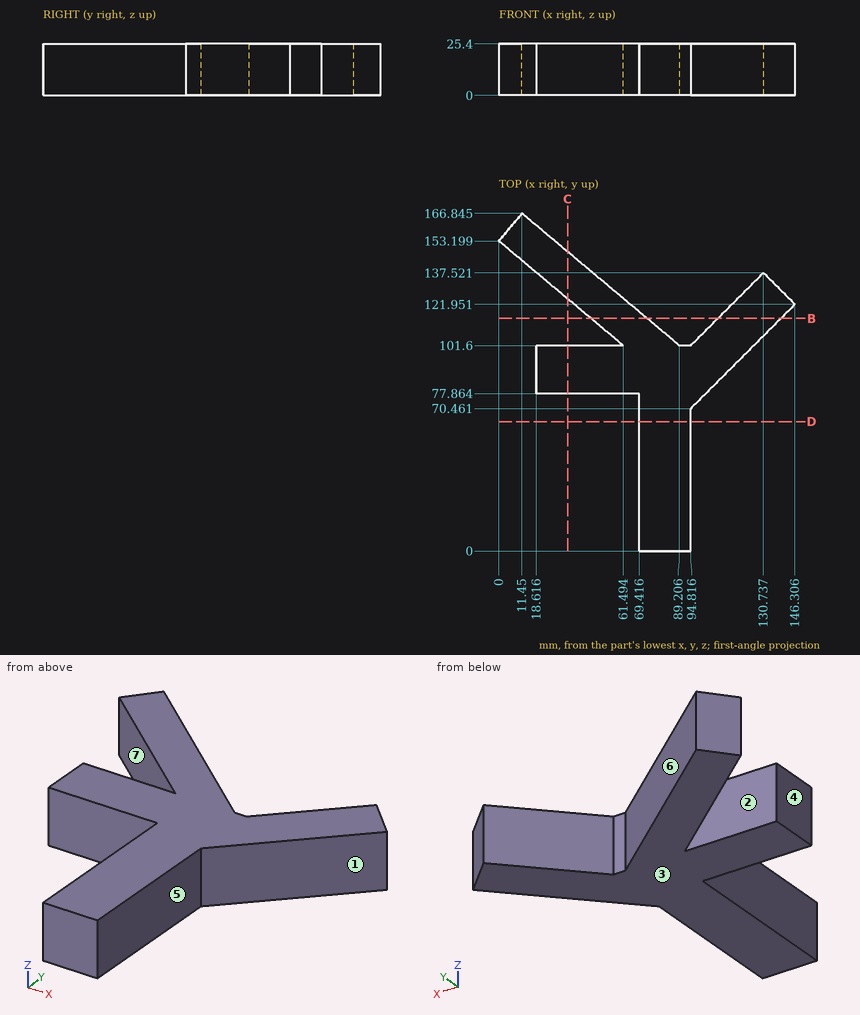
Check sheet for the drawn part. Datum: minimum x, y, z corner. Units: mm. A direction names the side the tool comes from. Round coordinates to 2 decimals unless told otherwise and drop trailing zeros. Loops run counter-clockwise (first coordinate to the right, second up) from the corner with the lowest first, then second, coordinate; pieces in that order, holes last. Notation, with made-up numbers: (47.25, 60) - (92.25, 60) arc R17 ccw to (92.25, 78) - close; hole circle Ø2 at (23.5, 36.5). An arc over 180 degrees is marked (long way). Write item = value, one per line. Start each with the question number.
1. Section check D-D on y = 64. Enter the section's corners in (x, z) (1 decimal).
2. Depth check by flat-ended pin: pin 1 (1 mm diameter, centred on x = 70.5, z = 17, fed in from +Y) (1 decimal); pin 2 (10 mm diameter, centred on y = 21, z = 7.5, fed in from +X); pin 3 (1 mm diameter, centred on y = 120.5, z = 5.5, fed in from +X) (1 decimal). Enter the tip coordinate at first touch or a pass-through.
3. Set-up check for the marked faces 4, 5, 6 and 7: record each of +Z, -Z, +X, -X, +Y, -Y from which the full face is reachable in a straight line by a thin tool's end or side.
4. Section check C-C on x = 34. Enter the section's corners in (y, z) (1 decimal), then the cut area to 3 significant figures.
5. Thickness scan on line 1 (Y direction, x = 60, z = 24.75) (1 decimal); line 2 (X direction, y = 135, z = 23) (1 decimal); line 3 (Y direction, x = 47.5, z = 15.25) (1 decimal). Record the ranges inside material, lowest first.
6. Section check B-B on y = 115. Enter the section's corners in (x, z) (1 decimal).
7. Mould release check, pull along Y, two halves, no side actions. Record for the marked faces 1, 2 and 3: released by +Y, released by -Y, zero draft, split by the parting line, or undercut.
Working result:
q1.outline = (69.4, 0) - (94.8, 0) - (94.8, 25.4) - (69.4, 25.4) - close
q2.pin_1 = 117.7
q2.pin_2 = 94.82
q2.pin_3 = 145.4
q3.face_4 = +Z, -Z, -X, -Y
q3.face_5 = +Z, -Z, +X, -Y
q3.face_6 = +Z, -Z, +Y
q3.face_7 = +Z, -Z, -X
q4.outline = (77.9, 0) - (101.6, 0) - (101.6, 25.4) - (77.9, 25.4) - close; (124.7, 0) - (147.9, 0) - (147.9, 25.4) - (124.7, 25.4) - close
q4.area = 1,190 mm^2
q5.line_1 = 77.9 to 101.6, 102.9 to 126.1
q5.line_2 = 21.7 to 49.4, 128.2 to 133.3
q5.line_3 = 77.9 to 101.6, 113.3 to 136.6
q6.outline = (45.5, 0) - (73.2, 0) - (73.2, 25.4) - (45.5, 25.4) - close; (108.2, 0) - (139.4, 0) - (139.4, 25.4) - (108.2, 25.4) - close
q7.face_1 = released by -Y
q7.face_2 = undercut
q7.face_3 = zero draft
